Input: dimensioned drawing with shaded views. Units: mm. Origin: part minimum x, y, z. A direction names the side the tool comes from. Coordinates: 2 decimals unless noted, no trailing zeros. Loops run counter-clockwise (first coordinate to the right, second up) from the corner with the lowest first, then second, coordinate; pieces in that order, holes last. Notation, with made-up numbers: (1.25, 15.25) -> (42.25, 15.25) arc R26 ccw to (42.25, 41.25) -> close; hole circle Ø2 at (2.25, -25.75). An arc over 180 degrees is marked (long way). Answer as CSV lines item,"result".
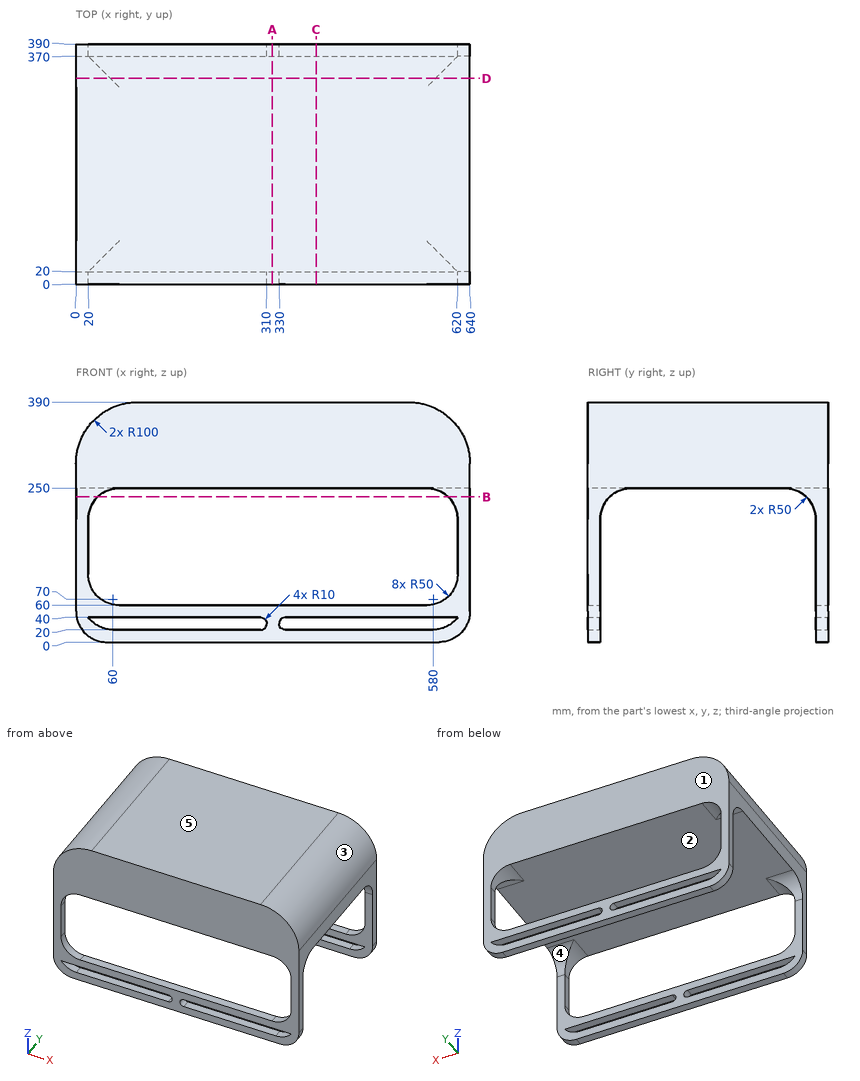
(1) Cut plane A-A (x = 319). Return the cut outline in (y, z), then the cut area to 3 significant figures.
Computed values:
outline,"(0, 0) -> (20, 0) -> (20, 60) -> (0, 60) -> close; (0, 250) -> (390, 250) -> (390, 390) -> (0, 390) -> close; (370, 0) -> (390, 0) -> (390, 60) -> (370, 60) -> close"
area,"57,000 mm^2"
(2) Pin query (flat end, axial travel): pin 1 Ø2 at (y, z) = (216, 350.5) entering from +X. Return the tip coordinate at first contact, or that it passes through.
Computed values:
pin 1,"x = 620.37"
(3) Draft query along X for the marked faces 1, 2 and 3. Return one class per face: released by +X, released by -X, zero draft, split by the parting line, or undercut.
Computed values:
face 1,"zero draft"
face 2,"undercut"
face 3,"released by +X"
(4) Material intervals for L1, parallel to Y at x = 51.5, z = 52; L2, parallel to Z at x = 224.5, y = 288; L3, parallel to X at y = 97, z = 365, sorted ascending. Write a range as [from, to].
Computed values:
L1,"[0, 20], [370, 390]"
L2,"[250, 390]"
L3,"[33.86, 606.14]"
(5) Cut plane B-B (z = 236). Return the cut outline in (x, y).
Computed values:
outline,"(0, 0) -> (35.3, 0) -> (35.3, 35.3) -> (0, 35.3) -> close; (0, 354.7) -> (35.3, 354.7) -> (35.3, 390) -> (0, 390) -> close; (604.7, 0) -> (640, 0) -> (640, 35.3) -> (604.7, 35.3) -> close; (604.7, 354.7) -> (640, 354.7) -> (640, 390) -> (604.7, 390) -> close"
(6) Access query for the marked faces 4 and 5. Directions: +Z, -Z, +X, -X, +Y, -Y. A direction counts if a zero-diameter tool reaches every point of the face in a straight line with its end or side. Return the directions, or none.
Computed values:
face 4,"-Z, +X, -X"
face 5,"+Z, +X, -X, +Y, -Y"
(7) Cut plane C-C (x = 390). Return the cut outline in (y, z).
Computed values:
outline,"(0, 0) -> (20, 0) -> (20, 20) -> (0, 20) -> close; (0, 40) -> (20, 40) -> (20, 60) -> (0, 60) -> close; (0, 250) -> (390, 250) -> (390, 390) -> (0, 390) -> close; (370, 0) -> (390, 0) -> (390, 20) -> (370, 20) -> close; (370, 40) -> (390, 40) -> (390, 60) -> (370, 60) -> close"
(8) Cut plane D-D (y = 334). Return the cut outline in (x, z).
Computed values:
outline,"(0, 248) -> (56, 248) arc R50 cw to (70, 250) -> (570, 250) arc R50 cw to (584, 248) -> (640, 248) -> (640, 290) arc R100 ccw to (540, 390) -> (100, 390) arc R100 ccw to (0, 290) -> close"
